Build history of the part. All positions in model axes, mm. Coordinates: 2 decimals unless noted, no trailing zeros. Write each loop counter-clockwise with the first axis right and the second up, starting at its lowest first coordinate (ties: lowest second). Pieces come first, ordered by that corner, then holes. Notation, with made-up numbers: (86.5, 78.25) -> (131.5, 78.25) arc R26 cw to (131.5, 102.25) -> close; hole circle Ø5 at (85, -37.75). An arc over 180 degrees is marked (long way). Write each question's results on one line, items separated by ' | '. Start each with the question number.
Q1. Saw through at B-B on y = -25. Give the cut face in (x, z).
Q2. Saw through at A-A on x = 0. Give the cut face in (y, z).
Q3. Saw through at C-C on z = -0.35. Give the cut face in (x, y) (3 decimals).
Q4. Saw through at D-D on y = -21.75. Give the cut face in (x, z), and give its area (3 significant figures).
Q5. Drop flat-ended pins along their axis: pin 1 Ø1 at (x, y) = (-0.5, -15) entering from -Z; pin 2 Ø1 at (y, z) = (-20, 0.5) entering from -X; pin 3 Ø1.6 at (x, y) = (0.5, -9) entering from +Z. Give the stop position or say it passes through.
Q6. Drill centre lines: line 1 (Y direction, x = 0, z = -0.5); line 2 (Y direction, x = -0.1, z = 1.3); line 3 (Y direction, x = -0.7, z = 0.95). Where is each one in solid material? Low to high.
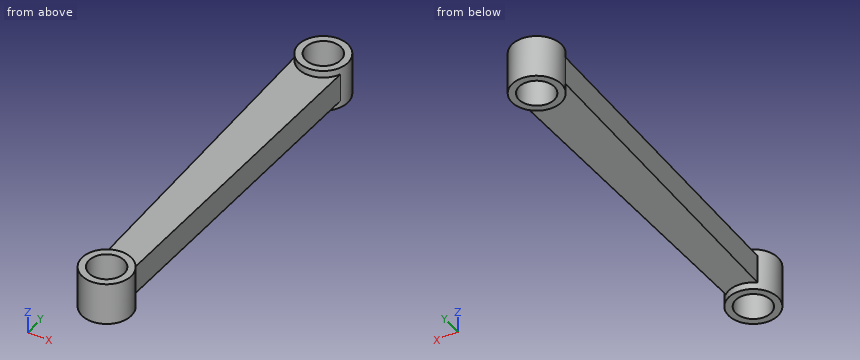
from build123d import *

# Parameters (mm, degrees)
SKETCH10_R                = 1.75
SKETCH10_R_2              = 1.25
BOSS_EXTRUDE1_DEPTH       = 1.5
BOSS_EXTRUDE1_DEPTH_BACK  = 1.5
SKETCH11_R                = 1.75
SKETCH11_R_2              = 1.25
BOSS_EXTRUDE12_DEPTH      = 1.5
BOSS_EXTRUDE12_DEPTH_BACK = 1.5
SKETCH1_R                 = 1.25
BOSS_EXTRUDE13_DEPTH      = 1
BOSS_EXTRUDE13_DEPTH_BACK = 1


with BuildPart() as part:
    # Sketch10 → Boss-Extrude1 (new body, two sides)
    with BuildSketch(Plane.XY) as boss_extrude1_sk:
        Circle(SKETCH10_R)
        Circle(SKETCH10_R_2, mode=Mode.SUBTRACT)
    extrude(amount=BOSS_EXTRUDE1_DEPTH)
    extrude(boss_extrude1_sk.sketch, amount=-BOSS_EXTRUDE1_DEPTH_BACK)



with BuildPart() as body_2:
    # Sketch11 → Boss-Extrude12 (new body, two sides)
    with BuildSketch(Plane.XY) as boss_extrude12_sk:
        with Locations((0, -25)):
            Circle(SKETCH11_R)
        with Locations((0, -25)):
            Circle(SKETCH11_R_2, mode=Mode.SUBTRACT)
    extrude(amount=BOSS_EXTRUDE12_DEPTH)
    extrude(boss_extrude12_sk.sketch, amount=-BOSS_EXTRUDE12_DEPTH_BACK)


with BuildPart() as part_1:
    add(part.part)

    add(body_2.part)  # Boss-Extrude13 merges body 2
    # Sketch1 → Boss-Extrude13 (add, two sides)
    with BuildSketch(Plane.XY) as boss_extrude13_sk:
        with BuildLine():
            Line((-1.625, -0.649519053), (-1.125, -23.659524338))
            ThreePointArc((-1.125, -23.659524338), (0, -26.75), (1.125, -23.659524338))
            Line((1.125, -23.659524338), (1.625, -0.649519053))
            ThreePointArc((1.625, -0.649519053), (0, 1.75), (-1.625, -0.649519053))
        make_face()
        Circle(SKETCH1_R, mode=Mode.SUBTRACT)
        with Locations((0, -25)):
            Circle(SKETCH1_R, mode=Mode.SUBTRACT)
    extrude(amount=BOSS_EXTRUDE13_DEPTH)
    extrude(boss_extrude13_sk.sketch, amount=-BOSS_EXTRUDE13_DEPTH_BACK)


solid = part_1.part
Returned:
1) outline: (-1.75, -1.5) -> (-1.25, -1.5) -> (-1.25, 1.5) -> (-1.75, 1.5) -> close; (1.25, -1.5) -> (1.75, -1.5) -> (1.75, 1.5) -> (1.25, 1.5) -> close
2) outline: (-26.75, -1.5) -> (-26.25, -1.5) -> (-26.25, 1.5) -> (-26.75, 1.5) -> close; (-23.75, -1.5) -> (-23.25, -1.5) -> (-23.25, -1) -> (-1.75, -1) -> (-1.75, -1.5) -> (-1.25, -1.5) -> (-1.25, 1.5) -> (-1.75, 1.5) -> (-1.75, 1) -> (-23.25, 1) -> (-23.25, 1.5) -> (-23.75, 1.5) -> close; (1.25, -1.5) -> (1.75, -1.5) -> (1.75, 1.5) -> (1.25, 1.5) -> close
3) outline: (-1.625, -0.65) -> (-1.125, -23.66) arc R1.75 ccw (long way) to (1.125, -23.66) -> (1.625, -0.65) arc R1.75 ccw (long way) to start; hole circle Ø2.5 at (0, -25); hole circle Ø2.5 at (0, 0)
4) outline: (-1.17, -1) -> (1.17, -1) -> (1.17, 1) -> (-1.17, 1) -> close | area: 4.67 mm2
5) pin 1: stops at z = -1 | pin 2: stops at x = -1.22 | pin 3: stops at z = 1
6) line 1: y = -26.75 to -26.25, -23.75 to -1.25, 1.25 to 1.75 | line 2: y = -26.75 to -26.25, -23.75 to -23.25, -1.75 to -1.25, 1.25 to 1.75 | line 3: y = -26.6 to -26.04, -23.96 to -1.04, 1.04 to 1.6
